Read the model definition and answer for the solid it produces. Units are mm, in the model's axes. Face numbers are marked on the shaded views. A direction names the side the tool comes from. Give positions to 0.01 mm unless a question says otherwise; leave off trailing zeros. Order: outer loops, then holes, each group sorted by start corner. A loop starts at its lowest first (then second) coordinate and runs counter-clockwise, first axis right, second up.
Item 1: Which of the six approach directions +Z, -Z, +X, -X, +Y, -Y give full straight-line access (tool end or side, diameter ignored) to the marked faces 1, 2 and 3?
Item 2: Given pin 1 Ø5 at (x, y) = (18, 0.5) entering from +Z; pin 2 Ø6 at (y, z) = (2.5, 39.5) entering from -X; pin 3 Ø2 at (y, z) = (2.5, 110) entering from -X, each flat-ended and moving along its own axis, determine where each tip first touches the part or whether it passes through.
Item 3: Find the intervals of material crossed by line 1 along Z through (x, y) = (55.5, 3.5); line 2 along X through (y, z) = (-1.5, 95); line 3 along Z through (x, y) = (-23, 4), in increasing order.
Item 4: A cutting plane is placed at A-A (x = 85.5). Write down the section's boundary in (y, z), plus the area to 3 significant figures.
Item 5: A cutting plane is placed at B-B (y = 2.5). Write down the section's boundary in (x, z), plus the area to 3 significant figures.
Item 6: A cutting plane is placed at C-C (z = 28.5). Write down the section's boundary in (x, y), plus the area to 3 significant figures.
Item 7: A cutting plane is placed at D-D (x = -17). Write down the section's boundary in (y, z), plus the area to 3 significant figures.
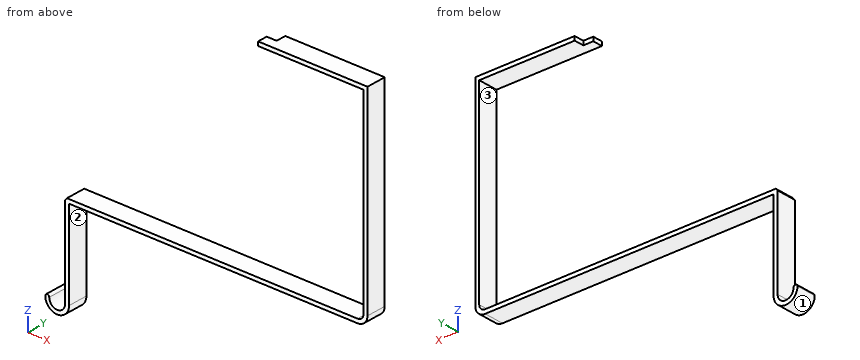
from build123d import *

# Parameters (mm, degrees)
F1_DEPTH = 5
F0_W     = 5
F0_H     = 2
F2_DEPTH = 5


# Not quite as in the source:
# - ends of sketch curves that miss each other by under 0.0002 mm in the source are joined


with BuildPart() as f1:
    # F0 (on Front) → F1 (new body, symmetric)
    with BuildSketch(Plane.XZ):
        with BuildLine():
            Line((103.7702985108, 110.5688567758), (53.7702985108, 110.5688567758))
            Line((53.7702985108, 110.5688567758), (53.7702985108, 108.5688567758))
            Line((53.7702985108, 108.5688567758), (101.7702985108, 108.5688567758))
            Line((101.7702985108, 108.5688567758), (101.7702985108, 11.5688567758))
            ThreePointArc((101.7702985108, 11.5688567758), (100.8916188543, 9.4475364322), (98.7702985108, 8.5688567758))
            Line((98.7702985108, 8.5688567758), (-47.322679311, 8.5688567758))
            Line((-47.322679311, 8.5688567758), (-48.2297014892, 7.4968221597))
            Line((-48.2297014892, 7.4968221597), (-48.2297014892, -37.4311432242))
            ThreePointArc((-48.2297014892, -37.4311432242), (-52.2297014892, -41.4311438799), (-56.2297021449, -37.4311432242))
            ThreePointArc((-56.2297021449, -37.4311432242), (-57.229701817, -36.4311435521), (-58.2297014892, -37.4311432242))
            ThreePointArc((-58.2297014892, -37.4311432242), (-52.2297014892, -43.4311432242), (-46.2297014892, -37.4311432242))
            Line((-46.2297014892, -37.4311432242), (-46.2297014892, 6.5688567758))
            Line((-46.2297014892, 6.5688567758), (98.7702985108, 6.5688567758))
            ThreePointArc((98.7702985108, 6.5688567758), (102.3058324167, 8.0333228698), (103.7702985108, 11.5688567758))
            Line((103.7702985108, 11.5688567758), (103.7702985108, 110.5688567758))
        make_face()
    extrude(amount=F1_DEPTH, both=True)

    # F0 (on Front) → F2 (join)
    with BuildSketch(Plane.XZ):
        with Locations((51.2702985108, 109.5688567758)):
            Rectangle(F0_W, F0_H)
    extrude(amount=F2_DEPTH)


solid = f1.part
Response values:
1. face 1: -Z, +Y, -Y
1. face 2: -Z, +X, +Y, -Y
1. face 3: -X, +Y, -Y
2. pin 1: stops at z = 8.57
2. pin 2: stops at x = 101.77
2. pin 3: stops at x = 53.77
3. line 1: z = 6.57 to 8.57, 108.57 to 110.57
3. line 2: x = 101.77 to 103.77
3. line 3: z = 6.57 to 8.57
4. outline: (-5, 6.57) - (5, 6.57) - (5, 8.57) - (-5, 8.57) - close; (-5, 108.57) - (5, 108.57) - (5, 110.57) - (-5, 110.57) - close
4. area: 40.0 mm2
5. outline: (-58.23, -37.43) arc R6 ccw to (-46.23, -37.43) - (-46.23, 6.57) - (98.77, 6.57) arc R5 ccw to (103.77, 11.57) - (103.77, 110.57) - (53.77, 110.57) - (53.77, 108.57) - (101.77, 108.57) - (101.77, 11.57) arc R3 cw to (98.77, 8.57) - (-47.32, 8.57) - (-48.23, 7.5) - (-48.23, -37.43) arc R4 cw to (-56.23, -37.43) arc R1 ccw to start
5. area: 721 mm2
6. outline: (101.77, -5) - (103.77, -5) - (103.77, 5) - (101.77, 5) - close
6. area: 20.0 mm2
7. outline: (-5, 6.57) - (5, 6.57) - (5, 8.57) - (-5, 8.57) - close
7. area: 20.0 mm2
